```python
from build123d import *

# Parameters (mm, degrees)
SK_TYRE_R               = 72
EX_TYRE_DEPTH           = 52
SK_RECESSDEEP_R         = 38
CUT_RECESSDEEP_DEPTH    = 32
CUT_RECESSSHALLOW_START = -16
SK_RECESSSHALLOW_R      = 38
CUT_RECESSSHALLOW_DEPTH = 16
SK_WEBHOLES_R           = 7
SK_WEBHOLES_R_2         = 2
CUT_WEBHOLES_DEPTH      = 4


with BuildPart() as part:
    # SK_Tyre → EX_Tyre (new body)
    with BuildSketch(Plane(origin=(-32, 0, 0), x_dir=(0, 0, -1), z_dir=(1, 0, 0))):
        Circle(SK_TYRE_R)
    extrude(amount=EX_TYRE_DEPTH)

    # SK_RecessDeep → CUT_RecessDeep (cut)
    with BuildSketch(Plane(origin=(-32, 0, 0), x_dir=(0, 0, -1), z_dir=(1, 0, 0))):
        Circle(SK_RECESSDEEP_R)
    extrude(amount=CUT_RECESSDEEP_DEPTH, mode=Mode.SUBTRACT)

    # SK_RecessShallow → CUT_RecessShallow (cut)
    with BuildSketch(Plane(origin=(20, 0, 0), x_dir=(0, 0, -1), z_dir=(1, 0, 0)).offset(CUT_RECESSSHALLOW_START)):
        Circle(SK_RECESSSHALLOW_R)
    extrude(amount=CUT_RECESSSHALLOW_DEPTH, mode=Mode.SUBTRACT)

    # SK_WebHoles → CUT_WebHoles (cut)
    with BuildSketch(Plane(origin=(0, 0, 0), x_dir=(0, 0, -1), z_dir=(1, 0, 0))):
        Circle(SK_WEBHOLES_R)
        with Locations((-8, 8)):
            Circle(SK_WEBHOLES_R_2)
        with Locations((-8, -8)):
            Circle(SK_WEBHOLES_R_2)
        with Locations((8, 8)):
            Circle(SK_WEBHOLES_R_2)
        with Locations((8, -8)):
            Circle(SK_WEBHOLES_R_2)
        with Locations((-16, 16)):
            Circle(SK_WEBHOLES_R_2)
        with Locations((-16, -16)):
            Circle(SK_WEBHOLES_R_2)
        with Locations((16, 16)):
            Circle(SK_WEBHOLES_R_2)
        with Locations((16, -16)):
            Circle(SK_WEBHOLES_R_2)
    extrude(amount=CUT_WEBHOLES_DEPTH, mode=Mode.SUBTRACT)


solid = part.part
```
Geometry check sheet. Reference: the model listing, model coordinates, mm. A direction names the side the tool comes from. Give positions to 0.01 mm unless a question says otherwise; leave off trailing zeros. Loops run counter-clockwise (first coordinate to the right, second up) from the corner with the lowest first, then second, coordinate; pieces in that order, holes last. Notation, with made-up numbers: M 33.5,-20.75 L 65.5,-20.75 A20 cw 65.5,8.25 Z; hole C 63,66.5 d2. An arc over 180 degrees is marked long. Answer as CSV lines item,"result".
Item 1: Cross-section at A-A on y = 0. Record the cut outline in (x, z).
Values:
outline,"M -32,-72 L 20,-72 L 20,-38 L 4,-38 L 4,-7 L 0,-7 L 0,-38 L -32,-38 Z; M -32,38 L 0,38 L 0,7 L 4,7 L 4,38 L 20,38 L 20,72 L -32,72 Z"
Item 2: Access from +Z, -Z, +X, -X, +Y, -Y to the whole of each face (thin tool, end or side, straight path). Record for faces 1 (the flat face through (4, -8, 1)), 2 (the flat face through (0, -8, 1)), 3 (the cylindrical face through (2, -14, 16)).
Values:
face 1,"+X"
face 2,"-X"
face 3,"+X, -X"
Item 3: Material ranges on line 1 (Y direction, x = 1.2, z = 8); line 2 (Y direction, x = -17, z = 0); line 3 (Y direction, x = 1.9, z = -16), recorded low to high.
Values:
line 1,"y = -71.55 to -10, -6 to 6, 10 to 71.55"
line 2,"y = -72 to -38, 38 to 72"
line 3,"y = -70.2 to -18, -14 to 14, 18 to 70.2"
Item 4: Cross-section at D-D on x = -6.5. Record the cut outline in (y, z).
Values:
outline,"C 0,0 d144; hole C 0,0 d76"
Item 5: Release check for a two-part mould opening along Z. For faces 4 (the cylindrical face through (2, -8, 10)), 5 (the cylindrical face through (-6.364, 71.387, 9.373)), 6 (the flat face through (-32, -31, -31)) record: pulls with the +Z half, pulls with the -Z half, needs draft (parallel to the pull), parting line crosses it, or undercut.
Values:
face 4,"undercut"
face 5,"parting line crosses it"
face 6,"needs draft"
Item 6: Cross-section at B-B on z = -16. Record the cut outline in (x, y), and give its area (3 significant figures).
Values:
outline,"M -32,-70.2 L 20,-70.2 L 20,-34.47 L 4,-34.47 L 4,-18 L 0,-18 L 0,-34.47 L -32,-34.47 Z; M -32,34.47 L 0,34.47 L 0,18 L 4,18 L 4,34.47 L 20,34.47 L 20,70.2 L -32,70.2 Z; M 0,-14 L 4,-14 L 4,14 L 0,14 Z"
area,"3,960 mm²"
Item 7: Depth check by flat-ended pin: P1, Ø2.5, axis at y = -16, z = -16, coming from the -X side; P2, Ø5, axis at x = -23.5, z = -16, coming from the +Y side; P3, Ø8, axis at x = -14, y = 57, coming from the +Z side; P4, Ø6.5, axis at y = 16, z = 16, coming from the -X side. Enter the tip coordinate at first touch or a pass-through.
Values:
P1,"passes through"
P2,"stops at y = 70.72"
P3,"stops at z = 48.73"
P4,"stops at x = 0"
